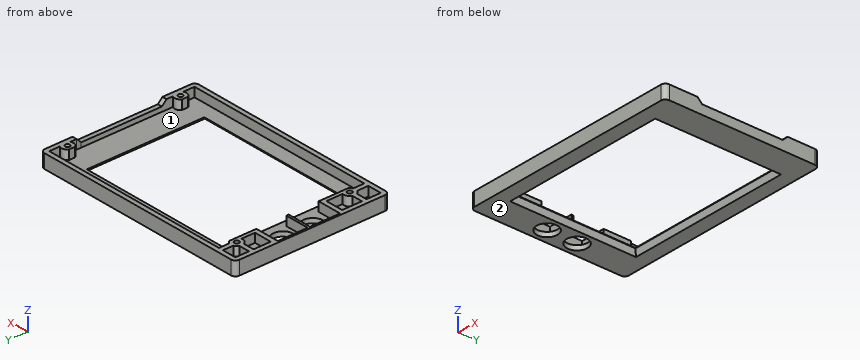
from build123d import *

# Parameters (mm, degrees)
SKETCH_2_R          = 4.5
SKETCH_2_W          = 67.8
SKETCH_2_H          = 51
EXTRUDE_1_DEPTH     = 2
SKETCH_3_R          = 1
EXTRUDE_2_DEPTH     = 4
SKETCH_4_W          = 7.723167142
SKETCH_4_H          = 2
SKETCH_4_W_2        = 2
SKETCH_4_H_2        = 9
SKETCH_4_H_3        = 10
EXTRUDE_3_DEPTH     = 3.8
CUT_EXTRUDE_1_DEPTH = 2
CHAMFER_2_SIZE      = 2
SKETCH_6_W          = 78.903110185
SKETCH_6_H          = 60.07500003
CUT_EXTRUDE_2_DEPTH = 4
CHAMFER_3_SIZE      = 1.8


with BuildPart() as part:
    # Эскиз2 → Бобышка-Вытянуть1 (new body)
    with BuildSketch(Plane.XY):
        with BuildLine():
            Line((-47.825, 31.6375), (-47.825, -31.6375))
            ThreePointArc((-47.825, -31.6375), (-47.268502884, -32.981002884), (-45.925, -33.5375))
            Line((-45.925, -33.5375), (45.925, -33.5375))
            ThreePointArc((45.925, -33.5375), (47.268502884, -32.981002884), (47.825, -31.6375))
            Line((47.825, -31.6375), (47.825, -19.36863872))
            Line((47.825, -19.36863872), (47.825, -17.36863872))
            Line((47.825, -17.36863872), (47.825, 17.677620675))
            Line((47.825, 17.677620675), (47.825, 19.677620675))
            Line((47.825, 19.677620675), (47.825, 31.6375))
            ThreePointArc((47.825, 31.6375), (47.268502884, 32.981002884), (45.925, 33.5375))
            Line((45.925, 33.5375), (-45.925, 33.5375))
            ThreePointArc((-45.925, 33.5375), (-47.268502884, 32.981002884), (-47.825, 31.6375))
        make_face()
        with Locations((-41.625, 7.212805211)):
            Circle(SKETCH_2_R, mode=Mode.SUBTRACT)
        with Locations((-41.625, -5.794271444)):
            Circle(SKETCH_2_R, mode=Mode.SUBTRACT)
        with Locations((0.165, 0.106266667)):
            Rectangle(SKETCH_2_W, SKETCH_2_H, mode=Mode.SUBTRACT)
    extrude(amount=EXTRUDE_1_DEPTH)

    # Эскиз3 → Бобышка-Вытянуть2 (add)
    with BuildSketch(Plane.XY.offset(2)):
        with BuildLine():
            ThreePointArc((47.825, 31.6375), (47.268502884, 32.981002884), (45.925, 33.5375))
            Line((45.925, 33.5375), (-45.925, 33.5375))
            ThreePointArc((-45.925, 33.5375), (-47.268502884, 32.981002884), (-47.825, 31.6375))
            Line((-47.825, 31.6375), (-47.825, -31.6375))
            ThreePointArc((-47.825, -31.6375), (-47.268502884, -32.981002884), (-45.925, -33.5375))
            Line((-45.925, -33.5375), (45.925, -33.5375))
            ThreePointArc((45.925, -33.5375), (47.268502884, -32.981002884), (47.825, -31.6375))
            Line((47.825, -31.6375), (47.825, 31.6375))
        make_face()
        with BuildLine():
            ThreePointArc((-41.101832747, -25.36863872), (-40.540310378, -26.207116351), (-39.701832747, -26.76863872))
            Line((-39.701832747, -26.76863872), (-39.701832747, -31.5375))
            Line((-39.701832747, -31.5375), (-45.825, -31.5375))
            Line((-45.825, -31.5375), (-45.825, -25.36863872))
            Line((-45.825, -25.36863872), (-41.101832747, -25.36863872))
        make_face(mode=Mode.SUBTRACT)
        with Locations((-38.701832747, -24.36863872)):
            Circle(SKETCH_3_R, mode=Mode.SUBTRACT)
        with BuildLine():
            ThreePointArc((-37.101832747, -22.319248567), (-39.361609166, -21.853744075), (-41.101832747, -23.36863872))
            Line((-41.101832747, -23.36863872), (-45.825, -23.36863872))
            Line((-45.825, -23.36863872), (-45.825, -13.994271444))
            Line((-45.825, -13.994271444), (-37.101832747, -13.994271444))
            Line((-37.101832747, -13.994271444), (-37.101832747, -22.319248567))
        make_face(mode=Mode.SUBTRACT)
        with Locations((44.601277438, -24.36863872)):
            Circle(SKETCH_3_R, mode=Mode.SUBTRACT)
        with BuildLine():
            Line((-36.101832858, 1.212805211), (-36.501832747, 1.212805211))
            Line((-36.501832747, 1.212805211), (-47.025, 1.212805211))
            Line((-47.025, 1.212805211), (-47.025, 14.212805211))
            Line((-47.025, 14.212805211), (-36.501832747, 14.212805211))
            Line((-36.501832747, 14.212805211), (-36.101832858, 14.212805211))
            Line((-36.101832858, 14.212805211), (-36.101832858, 24.677620706))
            ThreePointArc((-36.101832858, 24.677620706), (-36.538502092, 26.119841216), (-37.701832858, 27.077620706))
            Line((-37.701832858, 27.077620706), (-37.701832858, 31.53750003))
            Line((-37.701832858, 31.53750003), (45.824999889, 31.53750003))
            Line((45.824999889, 31.53750003), (45.824999889, 26.971635329))
            ThreePointArc((45.824999889, 26.971635329), (42.001277327, 24.677620706), (45.824999889, 22.383606083))
            Line((45.824999889, 22.383606083), (45.824999889, 19.677620706))
            Line((45.824999889, 19.677620706), (45.825, 17.677620675))
            Line((45.825, 17.677620675), (45.825, -17.36863872))
            Line((45.825, -17.36863872), (45.825, -19.36863872))
            Line((45.825, -19.36863872), (45.825, -22.074624097))
            ThreePointArc((45.825, -22.074624097), (42.001277438, -24.36863872), (45.825, -26.662653343))
            Line((45.825, -26.662653343), (45.825, -31.5375))
            Line((45.825, -31.5375), (-37.701832747, -31.5375))
            Line((-37.701832747, -31.5375), (-37.701832747, -26.76863872))
            ThreePointArc((-37.701832747, -26.76863872), (-36.538272941, -25.81051562), (-36.101832858, -24.367812827))
            Line((-36.101832858, -24.367812827), (-36.101832858, -12.794271444))
            Line((-36.101832858, -12.794271444), (-36.501832747, -12.794271444))
            Line((-36.501832747, -12.794271444), (-47.025, -12.794271444))
            Line((-47.025, -12.794271444), (-47.025, 0.205728556))
            Line((-47.025, 0.205728556), (-36.501832747, 0.205728556))
            Line((-36.501832747, 0.205728556), (-36.101832858, 0.205728556))
            Line((-36.101832858, 0.205728556), (-36.101832858, 1.212805211))
        make_face(mode=Mode.SUBTRACT)
        with BuildLine():
            Line((-45.825, 15.412805211), (-45.825, 23.677620675))
            Line((-45.825, 23.677620675), (-41.101832747, 23.677620675))
            ThreePointArc((-41.101832747, 23.677620675), (-39.361609166, 22.16272603), (-37.101832747, 22.628230522))
            Line((-37.101832747, 22.628230522), (-37.101832747, 15.412805211))
            Line((-37.101832747, 15.412805211), (-45.825, 15.412805211))
        make_face(mode=Mode.SUBTRACT)
        with Locations((-38.701832747, 24.677620675)):
            Circle(SKETCH_3_R, mode=Mode.SUBTRACT)
        with BuildLine():
            Line((-45.825, 25.677620675), (-45.825, 31.5375))
            Line((-45.825, 31.5375), (-39.701832747, 31.5375))
            Line((-39.701832747, 31.5375), (-39.701832747, 27.077620675))
            ThreePointArc((-39.701832747, 27.077620675), (-40.540310378, 26.516098306), (-41.101832747, 25.677620675))
            Line((-41.101832747, 25.677620675), (-45.825, 25.677620675))
        make_face(mode=Mode.SUBTRACT)
        with Locations((44.601277438, 24.677620675)):
            Circle(SKETCH_3_R, mode=Mode.SUBTRACT)
    extrude(amount=EXTRUDE_2_DEPTH)

    # Эскиз4 → Бобышка-Вытянуть3 (add)
    with BuildSketch(Plane.XY.offset(6)):
        with Locations((-41.963416429, 15.212805211)):
            Rectangle(SKETCH_4_W, SKETCH_4_H)
        with Locations((-37.101832858, 18.712805211)):
            Rectangle(SKETCH_4_W_2, SKETCH_4_H_2)
        with Locations((-41.963416429, -13.794271444)):
            Rectangle(SKETCH_4_W, SKETCH_4_H)
        with Locations((-37.101832858, -17.794271444)):
            Rectangle(SKETCH_4_W_2, SKETCH_4_H_3)
    extrude(amount=-EXTRUDE_3_DEPTH)

    # Эскиз5 → Вырез-Вытянуть1 (cut)
    with BuildSketch(Plane.XY.offset(6)):
        Polygon((47.825, -17.36863872), (47.825, -19.36863872), (45.825, -19.36863872), (45.825, -17.36863872), (45.825, 17.677620675), (45.824999889, 19.677620706), (47.825, 19.677620706), (47.825, 17.677620675), align=None)
    extrude(amount=-CUT_EXTRUDE_1_DEPTH, mode=Mode.SUBTRACT)

    # Фаска2
    chamfer_2_edges = [part.edges().sort_by_distance(p)[0] for p in [
        (46.824999945, 19.677620706, 4),
        (46.825, -19.36863872, 4),
    ]]
    chamfer(chamfer_2_edges, length=CHAMFER_2_SIZE - 0.0001)  # a hair under: the kernel refuses the full size

    # Эскиз6 → Вырез-Вытянуть2 (cut)
    with BuildSketch(Plane.XY.offset(2)):
        with Locations((2.949722235, 0.500000015)):
            Rectangle(SKETCH_6_W, SKETCH_6_H)
    extrude(amount=CUT_EXTRUDE_2_DEPTH, mode=Mode.SUBTRACT)

    # Фаска3
    chamfer_3_edges = [part.edges().sort_by_distance(p)[0] for p in [
        (34.065, 0.106266667, 0),
        (0.165, 25.606266667, 0),
        (-33.735, 0.106266667, 0),
        (0.165, -25.393733333, 0),
    ]]
    chamfer(chamfer_3_edges, length=CHAMFER_3_SIZE)


solid = part.part
Verification items for the finished model (mm, model axes). Face numbers are marked on the shaded views. Give positions to 0.01 mm unless a question says otherwise; leave off trailing zeros. Order: outer loops, then holes, each group sorted by start corner. A loop starts at its lowest first (then second) coordinate and runs counter-clockwise, first axis right, second up. Notation, with made-up numbers: (-14, 73.5) -> (31, 73.5) arc R23 ccw to (31, 95.5) -> close; hole circle Ø9 at (63, -14.5). An arc over 180 degrees is marked (long way). Answer as CSV lines item,"result".
Q1. Sectioned sample at C-C on y = 10. Record the cut outline in (x, z) (3 decimals).
Solutions:
outline,"(-47.825, 0) -> (-45.158, 0) -> (-45.158, 2) -> (-47.025, 2) -> (-47.025, 6) -> (-47.825, 6) -> close; (-38.092, 0) -> (-35.535, 0) -> (-33.735, 1.8) -> (-33.735, 2) -> (-38.092, 2) -> close; (34.065, 1.8) -> (35.865, 0) -> (47.825, 0) -> (47.825, 4) -> (45.825, 4) -> (45.825, 2) -> (34.065, 2) -> close"
Q2. Scan lines: probe 1 along X at (y, z) = (-24.5, 2.25) (1 decimal); probe 2 along X at (y, z) = (20.5, 4) (3 decimals); probe 3 along Y at (x, z) = (30, 4). Record each from-to range of solid material in increasing order.
Solutions:
probe 1,"x = -47.8 to -39.7, -37.7 to -36.5, 42.4 to 43.6, 45.6 to 47.8"
probe 2,"x = -47.825 to -45.825, -38.102 to -36.502, 45.825 to 47.825"
probe 3,"y = -33.54 to -31.54, 31.54 to 33.54"
Q3. Depth check by flat-ended pin: pin 1 (3 mm diameter, centred on x = -42.5, y = -28.5, fed in from +Z). Enter the tip coordinate at first touch or a pass-through.
Solutions:
pin 1,"stops at z = 2"
Q4. Release check for a two-part mould opening along X. For the marked faces 1 and 2 record: +X half, -X half, draft (parallel to the pull), parting line (faces both ways), or undercut.
Solutions:
face 1,"undercut"
face 2,"draft"
Q5. Sectioned sample at B-B on y = -20.5. Record the cut outline in (x, z) (3 decimals), plus the area to 3 significant figures.
Solutions:
outline,"(-47.825, 0) -> (-35.535, 0) -> (-33.735, 1.8) -> (-33.735, 2) -> (-36.502, 2) -> (-36.502, 6) -> (-38.102, 6) -> (-38.102, 2.2) -> (-37.102, 2.2) -> (-37.102, 2) -> (-45.825, 2) -> (-45.825, 6) -> (-47.825, 6) -> close; (34.065, 1.8) -> (35.865, 0) -> (47.825, 0) -> (47.825, 6) -> (45.825, 6) -> (45.825, 2) -> (34.065, 2) -> close"
area,"74.7 mm²"
Q6. Sectioned sample at A-A on x = -11. Record the cut outline in (y, z).
Solutions:
outline,"(-33.54, 0) -> (-27.19, 0) -> (-25.39, 1.8) -> (-25.39, 2) -> (-31.54, 2) -> (-31.54, 6) -> (-33.54, 6) -> close; (25.61, 1.8) -> (27.41, 0) -> (33.54, 0) -> (33.54, 6) -> (31.54, 6) -> (31.54, 2) -> (25.61, 2) -> close"
